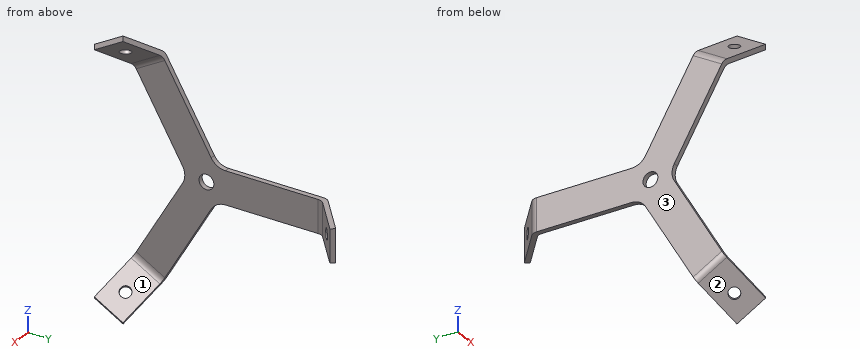
```python
from build123d import *

# Parameters (mm, degrees)
EXTRUDE_1_DEPTH          = 10
PATTERN_CIRCULAR_1_COUNT = 3
FILLET_2_R               = 10
HOLE_WIZARD_M82_D        = 9
HOLE_WIZARD_M61_D        = 6.6
PATTERN_CIRCULAR_2_COUNT = 3


with BuildPart() as part:
    # Sketch 1 → Extrude 1 (new, symmetric)
    with BuildSketch(Plane.XY):
        with BuildLine():
            Line((0, 0), (0, 69.067384684))
            ThreePointArc((0, 69.067384684), (0.468461065, 71.180475992), (1.786061952, 72.897606899))
            Line((1.786061952, 72.897606899), (24.052970465, 91.58176162))
            Line((24.052970465, 91.58176162), (25.981333294, 89.283628291))
            Line((25.981333294, 89.283628291), (4.786061952, 71.498683925))
            ThreePointArc((4.786061952, 71.498683925), (3.468461065, 69.781553018), (3, 67.668461709))
            Line((3, 67.668461709), (3, 0))
            Line((3, 0), (0, 0))
        make_face()
    extrude_1 = extrude(amount=EXTRUDE_1_DEPTH, both=True)

    # Pattern Circular 1: Extrude 1 ×3 about axis
    pattern_circular_1_axis = Axis((0, 0, 0), (1, 0, 0))
    for i in range(1, PATTERN_CIRCULAR_1_COUNT):
        add(extrude_1.rotate(pattern_circular_1_axis, i * 360 / PATTERN_CIRCULAR_1_COUNT))

    # Fillet 2
    fillet_2_edges = [part.edges().sort_by_distance(p)[0] for p in [
        (1.5, 5.773502692, 10),
        (1.5, 5.773502692, -10),
        (1.5, -11.547005384, 0),
    ]]
    fillet(fillet_2_edges, radius=FILLET_2_R)

    # Hole Wizard M82 (through all)
    with Locations(Plane(origin=(0, 0, 0), x_dir=(0, 0, -1), z_dir=(-1, 0, 0))):
        with Locations((0, 0)):
            Hole(HOLE_WIZARD_M82_D / 2)

    # Hole Wizard M61 (through all)
    with Locations(Plane(origin=(16.276728598, 81.14049807, 0), x_dir=(-0.766044443119, -0.642787609687, 0), z_dir=(0.642787609687, -0.766044443119, 0))):
        with Locations((0, 0)):
            hole_wizard_m61 = Hole(HOLE_WIZARD_M61_D / 2)

    # Pattern Circular 2: Hole Wizard M61 ×3 about axis
    pattern_circular_2_axis = Axis((22.676850282, 0, 0), (-1, 0, 0))
    for i in range(1, PATTERN_CIRCULAR_2_COUNT):
        add(hole_wizard_m61.rotate(pattern_circular_2_axis, i * 360 / PATTERN_CIRCULAR_2_COUNT), mode=Mode.SUBTRACT)


solid = part.part
```
Input: part model. Units: mm. Frame: model coordinates. Face numbers are marked on the shaded views. Coordinates: 2 decimals unless noted, no trailing zeros. Loops run counter-clockwise (first coordinate to the right, second up) from the corner with the lowest first, then second, coordinate; pieces in that order, holes last. Notation, with made-up numbers: M 4,63.25 L 38,63.25 A35 cw 38,101.25 Z; hole C 12,40 d2. An arc over 180 degrees is marked long. Answer in a Markdown table with one row per item.
1. Draft query along Z for the marked faces 1, 2 and 3. Return one class per face: pulls with the +Z half, pulls with the -Z half, needs draft (parallel to the pull), parting line crosses it, or undercut.
Response:
| item | result |
|---|---|
| face 1 | undercut |
| face 2 | pulls with the -Z half |
| face 3 | needs draft |
2. Section C-C, the plane x = 9.5. Output: boundary loops of the cut face in (y, z).
Response:
| item | result |
|---|---|
| outline | M -48.35,-63.74 L -31.02,-73.74 L -29.07,-70.35 L -46.39,-60.35 Z; M -48.35,63.74 L -46.39,60.35 L -29.07,70.35 L -31.02,73.74 Z; M 75.45,-10 L 79.37,-10 L 79.37,10 L 75.45,10 Z |
3. Section D-D, the plane y = 32.5. Output: boundary loops of the cut face in (x, z), then the cut area to 3 significant figures.
Response:
| item | result |
|---|---|
| outline | M 0,-10 L 3,-10 L 3,10 L 0,10 Z |
| area | 60.0 mm2 |
4. First-contact query: pin 1 (12 mm diameter, centred on x = 3, y = -25, fed in from +Z); pin 2 (6 mm diameter, centred on x = 3.5, z = 67, fed in from +Y). Flat tips, straight axial feed; report the tip coordinate or a pass-through.
Response:
| item | result |
|---|---|
| pin 1 | stops at z = 71.62 |
| pin 2 | stops at y = -25.43 |
5. Section A-A, the plane y = 0. Output: boundary loops of the cut face in (x, z).
Response:
| item | result |
|---|---|
| outline | M 0,-20 L 3,-20 L 3,-4.5 L 0,-4.5 Z; M 0,4.5 L 3,4.5 L 3,20 L 0,20 Z |
6. Section B-B, the plane z = 0. Output: boundary loops of the cut face in (x, y).
Response:
| item | result |
|---|---|
| outline | M 0,-13.09 L 3,-13.09 L 3,-4.5 L 0,-4.5 Z; M 0,4.5 L 3,4.5 L 3,67.67 A5 cw 4.79,71.5 L 13.75,79.02 L 11.82,81.32 L 1.79,72.9 A5 ccw 0,69.07 Z; M 16.88,85.56 L 18.8,83.26 L 25.98,89.28 L 24.05,91.58 Z |
7. Material intervals for line 1 (Y direction, x = 1, z = 0); line 2 (X direction, y = -21.5, z = -46); line 3 (Y direction, x = 2.1, z = 0), sorted ascending.
Response:
| item | result |
|---|---|
| line 1 | y = -13.09 to -4.5, 4.5 to 72.07 |
| line 2 | x = 0 to 3 |
| line 3 | y = -13.09 to -4.5, 4.5 to 73.16 |
